Verification items for the finished model (mm, model axes). A direction names the side the tool comes from. Round coordinates to 2 decimals unless told otherwise and drop trailing zeros. Write each loop counter-clockwise with the first axis right and the second up, starting at its lowest first coordinate (ties: lowest second). Pieces come first, ordered by that corner, then holes. Notation, with made-up numbers: M 18,-5.5 L 51,-5.5 A19 ccw 51,22.5 Z; hole C 40.5,8.25 d1. An arc over 180 degrees is marked long. Answer in a Markdown table with one row per item. Add a question column.
1. Draft check along Z on faces 3 (the flat face through (0, 0, 0)), 4 (the flat face through (1, 0, 3)), 5 (the flat face through (2, -3, 3)). Enter one of: pulls with the +Z half, pulls with the -Z half, needs draft (parallel to the pull), parting line crosses it, or undercut.
2. Sectioned sample at C-C on z = 3. Record the cut outline in (x, y), plus the area to 3 significant figures.
3. Material ranges on probe 1 along Y at (x, z) = (1.45, 3); probe 2 along Z at (x, y) = (2.5, 0.1); probe 3 along Z at (x, y) = (1.6, 1.25), recorded low to high.
4. Go/stop test with a flat-tipped pin: pin 1 Ø3 at (y, z) = (0, 3) entering from +X. Record where the tip stops, or that it passes through.
5. Sectioned sample at D-D on x = -2.5. Record the cut outline in (y, z).
6. Sectioned sample at B-B on y = 0. Record the cut outline in (x, z), plus the area to 3 significant figures.
7. Set-up check for faces 1 (the cylindrical face through (2.014, 0.496, 1.426)), 2 (the flat face through (0, 0, 6)): record each of +Z, -Z, +X, -X, +Y, -Y from which the full face is reachable in a straight line by a thin tool's end or side.
8. Sectioned sample at A-A on x = 1.65. Record the cut outline in (y, z), plus the area to 3 significant figures.
```python
from build123d import *

# Parameters (mm, degrees)
RESSALTO_EXTRUS_O1_DEPTH = 6
ESBO_O3_R                = 1.65
CORTE_EXTRUS_O1_DEPTH    = 2


with BuildPart() as part:
    # Esboço1 → Ressalto-extrusão1 (new body)
    with BuildSketch(Plane.XY):
        with BuildLine():
            Line((0, 3), (3, 3))
            Line((3, 3), (3, -3))
            Line((3, -3), (0, -3))
            ThreePointArc((0, -3), (-3, 0), (0, 3))
        make_face()
    extrude(amount=RESSALTO_EXTRUS_O1_DEPTH)

    # Esboço3 → Corte-extrusão1 (cut)
    with BuildSketch(Plane(origin=(3, 0, 0), x_dir=(0, 0, -1), z_dir=(1, 0, 0))):
        with Locations((-3, 0)):
            Circle(ESBO_O3_R)
    extrude(amount=-CORTE_EXTRUS_O1_DEPTH, mode=Mode.SUBTRACT)


solid = part.part
```
Geometry check:
| question | item | result |
|---|---|---|
| 1 | face 3 | pulls with the -Z half |
| 1 | face 4 | undercut |
| 1 | face 5 | needs draft |
| 2 | outline | M 0,-3 L 3,-3 L 3,-1.65 L 1,-1.65 L 1,1.65 L 3,1.65 L 3,3 L 0,3 A3 ccw Z |
| 2 | area | 25.5 mm2 |
| 3 | probe 1 | y = -3 to -1.65, 1.65 to 3 |
| 3 | probe 2 | z = 0 to 1.35, 4.65 to 6 |
| 3 | probe 3 | z = 0 to 1.92, 4.08 to 6 |
| 4 | pin 1 | stops at x = 1 |
| 5 | outline | M -1.66,0 L 1.66,0 L 1.66,6 L -1.66,6 Z |
| 6 | outline | M -3,0 L 3,0 L 3,1.35 L 1,1.35 L 1,4.65 L 3,4.65 L 3,6 L -3,6 Z |
| 6 | area | 29.4 mm2 |
| 7 | face 1 | +X |
| 7 | face 2 | +Z, +X, -X, +Y, -Y |
| 8 | outline | M -3,0 L 3,0 L 3,6 L -3,6 Z; hole C 0,3 d3.3 |
| 8 | area | 27.4 mm2 |
